Can you work these out from the drawing? Everything is in mm from the part's minimum corner. A direction names the side the tool comes from. Give positions to 0.01 mm unless a question says otherwise; leave off trailing zeros. Write each loop counter-clockwise with the first axis right and the second up, starting at its lowest first coordinate (ties: lowest second). Pieces come first, ordered by that corner, then holes. Notation, with made-up numbers: (-4, 40) -> (35, 40) arc R32 cw to (35, 78) -> close; hole circle Ø9 at (86, 57). An arc over 180 degrees is marked (long way). Use one line per item in the form item = value.
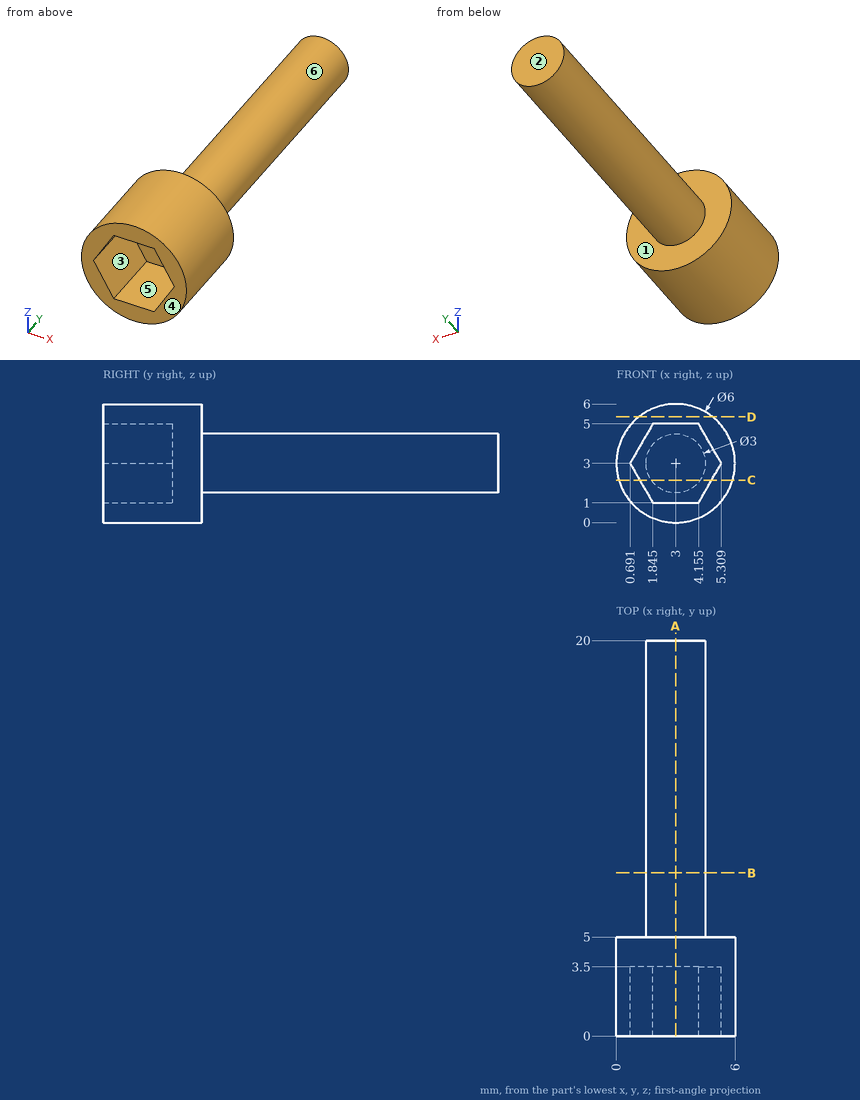
Q1. I want a section at C-C, the plane z = 2.15. Write out the boundary of the cut face in (x, y).
Result set:
outline = (0.12, 0) -> (1.18, 0) -> (1.18, 3.5) -> (4.82, 3.5) -> (4.82, 0) -> (5.88, 0) -> (5.88, 5) -> (4.24, 5) -> (4.24, 20) -> (1.76, 20) -> (1.76, 5) -> (0.12, 5) -> close
Q2. If I drill on line 1 along Z through (x, y) = (2.9, 1.75); line 2 along Y through (x, z) = (0.45, 1.95); line 3 along Y through (x, z) = (3.9, 3.8), over which ranges is the centre line in solid material (lowest first)? Write a range as from..to.
Result set:
line_1 = 0..1, 5..6
line_2 = 0..5
line_3 = 3.5..20
Q3. I want a section at D-D, the plane z = 5.35. Write out the boundary of the cut face in (x, y) (1 decimal).
Result set:
outline = (1.1, 0) -> (4.9, 0) -> (4.9, 5) -> (1.1, 5) -> close
Q4. I want a section at B-B, the plane y = 8.25. Write out the boundary of the cut face in (x, z).
Result set:
outline = circle Ø3 at (3, 3)
Q5. If we mould it in two halves opening along X, with no side actions, what happens to the marked faces 4, 5 and 6? For each: +X half, -X half, draft (parallel to the pull), parting line (faces both ways), or undercut.
Result set:
face_4 = draft
face_5 = undercut
face_6 = parting line
Q6. Will these pins go through, and if not, where does the flat tip stop? pin 1 Ø1.5 at (y, z) = (11.5, 2.5) entering from +X; pin 2 Ø1 at (x, y) = (2.5, 9) entering from +Z; pin 3 Ø1 at (x, y) = (2, 14) entering from -Z (1 decimal).
Result set:
pin_1 = 4.5
pin_2 = 4.5
pin_3 = 1.6
Q7. I want a section at A-A, the plane x = 3. Write out the boundary of the cut face in (y, z), and give its area (3 significant figures).
Result set:
outline = (0, 0) -> (5, 0) -> (5, 1.5) -> (20, 1.5) -> (20, 4.5) -> (5, 4.5) -> (5, 6) -> (0, 6) -> (0, 5) -> (3.5, 5) -> (3.5, 1) -> (0, 1) -> close
area = 61.0 mm2
Q8. Which directions (+Z, -Z, +X, -X, +Y, -Y) give clear straight access to the entire face, cutting with the end or side of a thin tool? Please do the marked faces 1, 2 and 3.
Result set:
face_1 = +Y
face_2 = +Z, -Z, +X, -X, +Y
face_3 = -Y
